Part model, mm, in its own coordinate system. Face numbers are marked on the shaded views. A direction names the side the tool comes from. Coordinates: 2 decimals unless noted, no trailing zeros. Write each loop counter-clockwise with the first axis right and the second up, starting at its lowest first coordinate (ties: lowest second). Pieces come first, ordered by that corner, then holes. Notation, with made-up numbers: M 56,-0.75 L 83,-0.75 A8 ccw 83,7.25 Z; hole C 4.5,17 d6. An arc over 180 degrees is marked long. Use a Markdown table: item, result. Add a question column.
Q1. Wall check: L1, parallel to Y at x = 0, z = 20.8 (3 decimals); L2, parallel to Z at x = -1.5, y = 3.75; L3, parallel to Z at x = -6, y = 0.1 (3 decimals). Give the ranges that are in metal, low to high. Write a range as from..to.
Q2. Pin check, flat tips, straight feed: pin 1 Ø1.6 at (x, z) = (4, 2.5) entering from +Y; pin 2 Ø0.6 at (x, z) = (5.5, 2.5) entering from -Y; pin 3 Ø1 at (y, z) = (1.5, 7.5) entering from -X. Stop position of each tip, or through.
Q3. Slice it at B-B on z = 2.5. Write the cut outline in (x, y) (3 decimals), then the cut area to 3 significant figures.
Q4. Slice it at A-A on y = 0. Write the cut outline in (x, z) (3 decimals), then the cut area to 3 significant figures.
Q5. Slice it at C-C on x = -6. Write the cut outline in (y, z) (3 decimals).
Q6. Slice it at D-D on x = 1.25. Write the cut outline in (y, z).
Q7. Mould opens along Y. For the marked faces 1, 2, 3 and 4 say: released by +Y, released by -Y, zero draft, split by the parting line, or undercut.
Q8. Tool access for the marked faces 5, 6, 7, 8 and 9: list every direction of +Z, -Z, +X, -X, +Y, -Y with a clear straight run to the whole face (end or side of a thin tool).
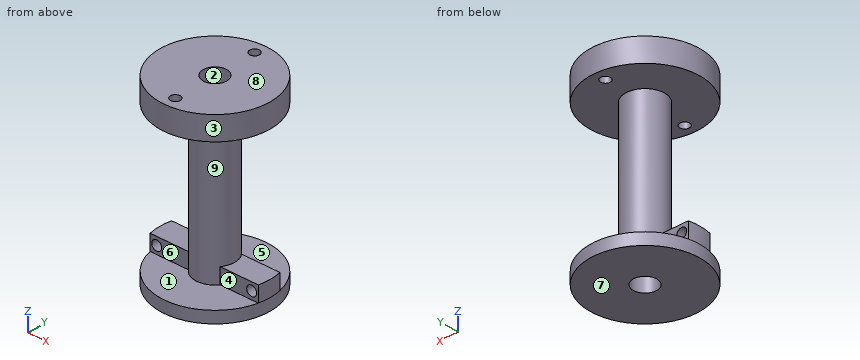
from build123d import *
from build123d.topology import SkipClean

# Parameters (mm, degrees)
SKETCH1_R           = 7
BOSS_EXTRUDE1_DEPTH = 1.5
SKETCH2_R           = 2.5
BOSS_EXTRUDE2_DEPTH = 18.5
SKETCH3_R           = 7
BOSS_EXTRUDE3_DEPTH = 3
CUT_EXTRUDE1_REACH  = 27.04
SKETCH4_R           = 1.5
CUT_EXTRUDE4_REACH  = 27.04
SKETCH5_R           = 0.625
BOSS_EXTRUDE5_DEPTH = 2
CUT_EXTRUDE5_REACH  = 27.5
SKETCH16_R          = 0.625
CUT_EXTRUDE6_REACH  = 25.67
SKETCH17_R          = 1.5


with BuildPart() as part:
    # Sketch1 → Boss-Extrude1 (new body)
    with BuildSketch(Plane.XY):
        Circle(SKETCH1_R)
    extrude(amount=BOSS_EXTRUDE1_DEPTH)

    # Sketch2 → Boss-Extrude2 (add)
    with BuildSketch(Plane.XY.offset(1.5)):
        Circle(SKETCH2_R)
    extrude(amount=BOSS_EXTRUDE2_DEPTH)

    # Sketch3 → Boss-Extrude3 (add)
    with BuildSketch(Plane.XY.offset(20)):
        Circle(SKETCH3_R)
    extrude(amount=BOSS_EXTRUDE3_DEPTH)

    # Sketch4 → Cut-Extrude1 (cut, up to next)
    with BuildSketch(Plane(origin=(0, 0, 0), x_dir=(-1, 0, 0), z_dir=(0, 0, -1)), mode=Mode.PRIVATE) as cut_extrude1_sk1:
        Circle(SKETCH4_R)
    cut_extrude1_tool1 = extrude(cut_extrude1_sk1.sketch, amount=-CUT_EXTRUDE1_REACH, mode=Mode.PRIVATE) & part.part
    add(cut_extrude1_tool1.solids().sort_by_distance((0, 0, 0))[0], mode=Mode.SUBTRACT)

    # Sketch5 → Cut-Extrude4 (cut, up to next)
    with BuildSketch(Plane.XY.offset(23), mode=Mode.PRIVATE) as cut_extrude4_sk1:
        with Locations((0, 5.5)):
            Circle(SKETCH5_R)
    cut_extrude4_tool1 = extrude(cut_extrude4_sk1.sketch, amount=-CUT_EXTRUDE4_REACH, mode=Mode.PRIVATE) & part.part
    # Sketch5 → Cut-Extrude4 (cut, up to next)
    with BuildSketch(Plane.XY.offset(23), mode=Mode.PRIVATE) as cut_extrude4_sk2:
        with Locations((0, -5.5)):
            Circle(SKETCH5_R)
    cut_extrude4_tool2 = extrude(cut_extrude4_sk2.sketch, amount=-CUT_EXTRUDE4_REACH, mode=Mode.PRIVATE) & part.part
    add(cut_extrude4_tool1.solids().sort_by_distance((0, 5.5, 23))[0], mode=Mode.SUBTRACT)
    add(cut_extrude4_tool2.solids().sort_by_distance((0, -5.5, 23))[0], mode=Mode.SUBTRACT)

    # Sketch15 → Boss-Extrude5 (add)
    with SkipClean():  # the faces are left unmerged after this step: merging them gives an invalid solid
        with BuildSketch(Plane.XY.offset(1.5)):
            with BuildLine():
                Line((6.837397, -1.5), (-6.837397, -1.5))
                ThreePointArc((-6.837397, -1.5), (-7, 0), (-6.837397, 1.5))
                Line((-6.837397, 1.5), (6.837397, 1.5))
                ThreePointArc((6.837397, 1.5), (7, 0), (6.837397, -1.5))
            make_face()
        extrude(amount=BOSS_EXTRUDE5_DEPTH)

    # Sketch16 → Cut-Extrude5 (cut, up to next)
    with BuildSketch(Plane.XZ.offset(1.5), mode=Mode.PRIVATE) as cut_extrude5_sk1:
        with Locations((-6, 2.5)):
            Circle(SKETCH16_R)
    cut_extrude5_tool1 = extrude(cut_extrude5_sk1.sketch, amount=-CUT_EXTRUDE5_REACH, mode=Mode.PRIVATE) & part.part
    # Sketch16 → Cut-Extrude5 (cut, up to next)
    with BuildSketch(Plane.XZ.offset(1.5), mode=Mode.PRIVATE) as cut_extrude5_sk2:
        with Locations(Location((6, 2.5, 0), (0, 0, 270))):
            Circle(SKETCH16_R)
    cut_extrude5_tool2 = extrude(cut_extrude5_sk2.sketch, amount=-CUT_EXTRUDE5_REACH, mode=Mode.PRIVATE) & part.part
    add(cut_extrude5_tool1.solids().sort_by_distance((-6, -1.5, 2.5))[0], mode=Mode.SUBTRACT)
    add(cut_extrude5_tool2.solids().sort_by_distance((6, -1.5, 2.5))[0], mode=Mode.SUBTRACT)

    # Sketch17 → Cut-Extrude6 (cut, up to next)
    with BuildSketch(Plane(origin=(0, 0, 1.5), x_dir=(-1, 0, 0), z_dir=(0, 0, -1)), mode=Mode.PRIVATE) as cut_extrude6_sk1:
        Circle(SKETCH17_R)
    cut_extrude6_tool1 = extrude(cut_extrude6_sk1.sketch, amount=-CUT_EXTRUDE6_REACH, mode=Mode.PRIVATE) & part.part
    add(cut_extrude6_tool1.solids().sort_by_distance((0, 0, 1.5))[0], mode=Mode.SUBTRACT)


solid = part.part
Recorded:
| question | item | result |
|---|---|---|
| 1 | L1 | -7..-6.125, -4.875..-1.5, 1.5..4.875, 6.125..7 |
| 1 | L2 | 0..1.5, 20..23 |
| 1 | L3 | 0..1.875, 3.125..3.5, 20..23 |
| 2 | pin 1 | y = 1.5 |
| 2 | pin 2 | y = -1.5 |
| 2 | pin 3 | x = -2.29 |
| 3 | outline | M -6.837,-1.5 L -6.625,-1.5 L -6.625,1.5 L -6.837,1.5 A7 ccw Z; M -5.375,-1.5 L -2,-1.5 A2.5 ccw 2,-1.5 L 5.375,-1.5 L 5.375,1.5 L 2,1.5 A2.5 ccw -2,1.5 L -5.375,1.5 Z; M 6.625,-1.5 L 6.837,-1.5 A7 ccw 6.837,1.5 L 6.625,1.5 Z; hole C 0,0 d3 |
| 3 | area | 32.7 mm² |
| 4 | outline | M -7,0 L -1.5,0 L -1.5,23 L -7,23 L -7,20 L -2.5,20 L -2.5,3.5 L -7,3.5 Z; M 1.5,0 L 7,0 L 7,3.5 L 2.5,3.5 L 2.5,20 L 7,20 L 7,23 L 1.5,23 Z; hole C -6,2.5 d1.25; hole C 6,2.5 d1.25 |
| 4 | area | 102 mm² |
| 5 | outline | M -3.606,0 L 3.606,0 L 3.606,1.5 L 1.5,1.5 L 1.5,1.875 L -1.5,1.875 L -1.5,1.5 L -3.606,1.5 Z; M -3.606,20 L 3.606,20 L 3.606,23 L -3.606,23 Z; M -1.5,3.125 L 1.5,3.125 L 1.5,3.5 L -1.5,3.5 Z |
| 6 | outline | M -6.89,0 L -0.83,0 L -0.83,23 L -6.89,23 L -6.89,20 L -2.17,20 L -2.17,1.5 L -6.89,1.5 Z; M 0.83,0 L 6.89,0 L 6.89,1.5 L 2.17,1.5 L 2.17,20 L 6.89,20 L 6.89,23 L 0.83,23 Z |
| 7 | face 1 | zero draft |
| 7 | face 2 | undercut |
| 7 | face 3 | split by the parting line |
| 7 | face 4 | released by -Y |
| 8 | face 5 | +Y |
| 8 | face 6 | -X, -Y |
| 8 | face 7 | -Z, +X, -X, +Y, -Y |
| 8 | face 8 | +Z, +X, -X, +Y, -Y |
| 8 | face 9 | none |
